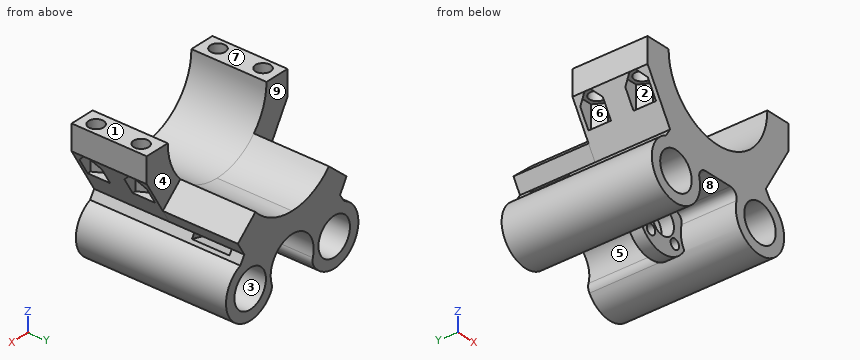
```python
from build123d import *

# Parameters (mm, degrees)
SKETCH1_R           = 11.5
SKETCH1_R_2         = 7.5
BOSS_EXTRUDE1_DEPTH = 30
FILLET1_R           = 3
SKETCH2_R           = 11.75
CUT_EXTRUDE3_DEPTH  = 3
SKETCH3_R           = 11.75
SKETCH3_R_2         = 5.25
SKETCH3_R_3         = 2
BOSS_EXTRUDE2_DEPTH = 5
SKETCH4_W           = 40
SKETCH4_H           = 60
BOSS_EXTRUDE3_DEPTH = 2
SKETCH5_R           = 10.25
CUT_EXTRUDE4_DEPTH  = 27
FILLET2_START       = -3
FILLET2_DEPTH       = 34
BOSS_EXTRUDE4_DEPTH = 30
BOSS_EXTRUDE5_DEPTH = 30
CUT_EXTRUDE5_DEPTH  = 15
SKETCH9_R           = 3
CUT_EXTRUDE6_DEPTH  = 10
CUT_EXTRUDE7_DEPTH  = 10


with BuildPart() as part:
    # Sketch1 → Boss-Extrude1 (new, symmetric)
    # profile 1 of 3: a face of its own
    with BuildSketch(Plane(origin=(0, 0, 0), x_dir=(1, 0, 0), z_dir=(0, 1, 0))):
        with Locations((-20, 0)):
            Circle(SKETCH1_R)
        with Locations(Location((-20, 0, 0), (0, 0, 270))):
            Circle(SKETCH1_R_2, mode=Mode.SUBTRACT)
    # profile 2 of 3: a face of its own
    with BuildSketch(Plane(origin=(0, 0, 0), x_dir=(1, 0, 0), z_dir=(0, 1, 0))):
        with Locations((20, 0)):
            Circle(SKETCH1_R)
        with Locations(Location((20, 0, 0), (0, 0, 270))):
            Circle(SKETCH1_R_2, mode=Mode.SUBTRACT)
    # profile 3 of 3: a face of its own
    with BuildSketch(Plane(origin=(0, 0, 0), x_dir=(1, 0, 0), z_dir=(0, 1, 0))):
        with BuildLine():
            ThreePointArc((-10.513167019, -6.5), (-14.638097353, -10.173494975), (-20, -11.5))
            Line((-20, -11.5), (20, -11.5))
            ThreePointArc((20, -11.5), (14.638097353, -10.173494975), (10.513167019, -6.5))
            Line((10.513167019, -6.5), (-10.513167019, -6.5))
        make_face()
    extrude(amount=BOSS_EXTRUDE1_DEPTH, both=True)

    # Fillet1
    fillet1_edges = [part.edges().sort_by_distance(p)[0] for p in [
        (-10.513167019, 0, 6.5),
        (10.513167019, 0, 6.5),
    ]]
    fillet(fillet1_edges, radius=FILLET1_R)

    # Sketch2 → Cut-Extrude3 (cut, symmetric)
    with BuildSketch(Plane(origin=(0, 0, 0), x_dir=(1, 0, 0), z_dir=(0, 1, 0))):
        Circle(SKETCH2_R)
    extrude(amount=CUT_EXTRUDE3_DEPTH, both=True, mode=Mode.SUBTRACT)

    # Sketch3 → Boss-Extrude2 (add)
    with BuildSketch(Plane(origin=(0, -3, 0), x_dir=(1, 0, 0), z_dir=(0, 1, 0))):
        Circle(SKETCH3_R)
        with Locations(Location((0, 0, 0), (0, 0, 270))):
            Circle(SKETCH3_R_2, mode=Mode.SUBTRACT)
        with Locations(Location((5.656854249, 5.656854249, 0), (0, 0, 270))):
            Circle(SKETCH3_R_3, mode=Mode.SUBTRACT)
        with Locations(Location((-5.656854249, 5.656854249, 0), (0, 0, 270))):
            Circle(SKETCH3_R_3, mode=Mode.SUBTRACT)
    extrude(amount=-BOSS_EXTRUDE2_DEPTH)

    # Sketch4 → Boss-Extrude3 (add)
    with BuildSketch(Plane.XY.offset(11.5)):
        Rectangle(SKETCH4_W, SKETCH4_H)
    extrude(amount=BOSS_EXTRUDE3_DEPTH)

    # Chamfer1
    # the kernel refuses this chamfer: 8 mm, written as the material it adds along each edge
    with BuildSketch(Plane(origin=(20, -30, 11.5), x_dir=(0.9777449098895067, 0, -0.20979726210120203), z_dir=(0, 1, 0))) as chamfer1_piece_1_section:
        with BuildLine():
            Line((5.051611198, 0.22627417), (-1.544518324, -6.369855352))
            Line((-1.544518324, -6.369855352), (-1.70095751, -6.33628779))
            ThreePointArc((-1.70095751, -6.33628779), (-0.843748586, -3.169588005), (-0.156439186, 0.033567562))
            Line((-0.156439186, 0.033567562), (0.033567562, 0.156439186))
            ThreePointArc((0.033567562, 0.156439186), (2.527924683, -0.095347808), (5.018043636, 0.382713356))
            Line((5.018043636, 0.382713356), (5.051611198, 0.22627417))
        make_face()
    chamfer1_piece_1 = extrude(amount=60, mode=Mode.PRIVATE)
    chamfer1_piece_1 = split(chamfer1_piece_1, bisect_by=Plane(origin=(20, -30, 13.5), z_dir=(0, 0, -1)), keep=Keep.TOP, mode=Mode.PRIVATE)
    add(chamfer1_piece_1)
    with BuildSketch(Plane(origin=(-20, -30, 11.5), x_dir=(-0.9777449098895067, 0, -0.20979726210120223), z_dir=(0, 1, 0))) as chamfer1_piece_2_section:
        with BuildLine():
            Line((5.051611198, -0.22627417), (-1.544518324, 6.369855352))
            Line((-1.544518324, 6.369855352), (-1.70095751, 6.33628779))
            ThreePointArc((-1.70095751, 6.33628779), (-0.843748586, 3.169588005), (-0.156439186, -0.033567562))
            Line((-0.156439186, -0.033567562), (0.033567562, -0.156439186))
            ThreePointArc((0.033567562, -0.156439186), (2.527924683, 0.095347808), (5.018043636, -0.382713356))
            Line((5.018043636, -0.382713356), (5.051611198, -0.22627417))
        make_face()
    chamfer1_piece_2 = extrude(amount=60, mode=Mode.PRIVATE)
    chamfer1_piece_2 = split(chamfer1_piece_2, bisect_by=Plane(origin=(-20, -30, 13.5), z_dir=(0, 0, -1)), keep=Keep.TOP, mode=Mode.PRIVATE)
    add(chamfer1_piece_2)

    # Sketch5 → Cut-Extrude4 (cut)
    with BuildSketch(Plane(origin=(0, 30, 0), x_dir=(1, 0, 0), z_dir=(0, 1, 0))):
        Circle(SKETCH5_R)
    extrude(amount=-CUT_EXTRUDE4_DEPTH, mode=Mode.SUBTRACT)

    # Fillet2: read off the stored shape, not the designer's step
    # Fillet2 outline → Fillet2 (cut)
    with BuildSketch(Plane(origin=(0, 0, 0), x_dir=(1, 0, 0), z_dir=(0, 1, 0)).offset(FILLET2_START)):
        with BuildLine():
            ThreePointArc((-9.833031798, 2.893783968), (-9.601199579, 3.588797381), (-9.3203125, 4.265474757))
            ThreePointArc((-9.3203125, 4.265474757), (-9.763069468, 5.239776072), (-10.294479167, 6.168700459))
            ThreePointArc((-10.294479167, 6.168700459), (-9.709438477, 4.581166738), (-9.833031798, 2.893783968))
        make_face()
        with BuildLine():
            ThreePointArc((10.294479167, 6.168700459), (9.763069468, 5.239776072), (9.3203125, 4.265474757))
            ThreePointArc((9.3203125, 4.265474757), (9.601199579, 3.588797381), (9.833031798, 2.893783968))
            ThreePointArc((9.833031798, 2.893783968), (9.709438477, 4.581166738), (10.294479167, 6.168700459))
        make_face()
    extrude(amount=FILLET2_DEPTH, mode=Mode.SUBTRACT)

    # Sketch6 → Boss-Extrude4 (add)
    with BuildSketch(Plane.XZ.offset(30)):
        with BuildLine():
            ThreePointArc((-23.5, 42), (0, 18.5), (23.5, 42))
            Line((23.5, 42), (33.5, 42))
            Line((33.5, 42), (33.5, 32))
            Line((33.5, 32), (22.769957826, 13.5))
            Line((22.769957826, 13.5), (-22.769957826, 13.5))
            Line((-22.769957826, 13.5), (-33.5, 32))
            Line((-33.5, 32), (-33.5, 42))
            Line((-33.5, 42), (-23.5, 42))
        make_face()
    extrude(amount=-BOSS_EXTRUDE4_DEPTH)

    # Sketch7 → Boss-Extrude5 (add)
    with BuildSketch(Plane(origin=(0, 0, 0), x_dir=(1, 0, 0), z_dir=(0, 1, 0))):
        with BuildLine():
            Line((0, -13.5), (0, -18.5))
            ThreePointArc((0, -18.5), (9.582977152, -20.542680761), (17.5, -26.315612859))
            Line((17.5, -26.315612859), (25.858213649, -18.824558077))
            Line((25.858213649, -18.824558077), (22.769957826, -13.5))
            Line((22.769957826, -13.5), (0, -13.5))
        make_face()
        with BuildLine():
            Line((-22.769957826, -13.5), (-25.858213649, -18.824558077))
            Line((-25.858213649, -18.824558077), (-17.5, -26.315612859))
            ThreePointArc((-17.5, -26.315612859), (-9.582977152, -20.542680761), (0, -18.5))
            Line((0, -18.5), (0, -13.5))
            Line((0, -13.5), (-22.769957826, -13.5))
        make_face()
    extrude(amount=BOSS_EXTRUDE5_DEPTH)

    # Sketch8 → Cut-Extrude5 (cut)
    with BuildSketch(Plane(origin=(0, 25, 0), x_dir=(1, 0, 0), z_dir=(0, 1, 0))):
        with BuildLine():
            Line((30.953633553, -14.257784453), (29.292282812, -15.746771207))
            ThreePointArc((29.292282812, -15.746771207), (0, -10.191127392), (-29.292282812, -15.746771207))
            Line((-29.292282812, -15.746771207), (-30.953633553, -14.257784453))
            ThreePointArc((-30.953633553, -14.257784453), (0, -8.191127392), (30.953633553, -14.257784453))
        make_face()
    extrude(amount=-CUT_EXTRUDE5_DEPTH, mode=Mode.SUBTRACT)

    # Sketch9 → Cut-Extrude6 (cut)
    with BuildSketch(Plane.XY.offset(42)):
        with Locations((29, -6)):
            Circle(SKETCH9_R)
        with Locations(Location((-29, -6, 0), (0, 0, 180))):
            Circle(SKETCH9_R)
        with Locations((-29, -24)):
            Circle(SKETCH9_R)
        with Locations(Location((29, -24, 0), (0, 0, 180))):
            Circle(SKETCH9_R)
    extrude(amount=-CUT_EXTRUDE6_DEPTH, mode=Mode.SUBTRACT)

    # Sketch10 → Cut-Extrude7 (cut)
    with BuildSketch(Plane.XY.offset(32)):
        Polygon((34.196152423, -6), (31.598076211, -1.5), (26.401923789, -1.5), (23.803847577, -6), (26.401923789, -10.5), (31.598076211, -10.5), align=None)
        Polygon((31.598076211, -19.5), (34.196152423, -24), (31.598076211, -28.5), (26.401923789, -28.5), (23.803847577, -24), (26.401923789, -19.5), align=None)
        Polygon((-34.196152423, -24), (-31.598076211, -28.5), (-26.401923789, -28.5), (-23.803847577, -24), (-26.401923789, -19.5), (-31.598076211, -19.5), align=None)
        Polygon((-31.598076211, -10.5), (-34.196152423, -6), (-31.598076211, -1.5), (-26.401923789, -1.5), (-23.803847577, -6), (-26.401923789, -10.5), align=None)
    extrude(amount=-CUT_EXTRUDE7_DEPTH, mode=Mode.SUBTRACT)


solid = part.part
```
The listing builds one solid part. Answer for the finished solid, in the listing's coordinates (mm). Face numbers are marked on the shaded views. A direction names the side the tool comes from. Round coordinates to 2 decimals unless told otherwise and drop trailing zeros. Write each loop counter-clockwise with the first axis right and the second up, starting at its lowest first coordinate (ties: lowest second). Pieces come first, ordered by that corner, then holes. Notation, with made-up numbers: (-34.5, -18.5) -> (-27.5, -18.5) arc R25 cw to (-27.5, -0.5) -> close; hole circle Ø3 at (-8.5, 25.25). An arc over 180 degrees is marked (long way). Answer as a JSON object with one key per item and string values. Group by question number.
Q1. Section D-D (z = 21) is taken. Write down the section's boundary in (x, y), plus the area to 3 significant figures.
Q2. Straight lines are drawn through the part: line 1 along Y through (x, z) = (29, 37); line 2 along X through (y, z) = (-18, 0); line 3 along X through (y, z) = (-7, 0). For each, find the intervals that lie inside material, in ascending order.
Q3. Determine the mould class of the marked faces 6, 7, 8 and 9 for opening direction Z: pulls with the +Z half, pulls with the -Z half, needs draft (parallel to the pull), parting line crosses it, or undercut.
Q4. Which of the six approach directions +Z, -Z, +X, -X, +Y, -Y give full straight-line access (tool end or side, diameter ignored) to the marked faces 1, 2, 3, 4 and 5?
Q5. Each of these flat-tipped pins is pushed along its axis until it touches: pin 1 Ø10 at (x, z) = (-21, 1.5) entering from -Y; pin 2 Ø16.5 at (x, z) = (0, 0) entering from +Y; pin 3 Ø8 at (y, z) = (10.5, -2) entering from -X; pin 4 Ø10 at (x, y) = (-25.5, 11.5) entering from -Z. Where does it stop, or does it pass through?
Q6. Section A-A (z = 34) is taken. Write down the section's boundary in (x, y).
Q7. Section B-B (x = -14) is taken. Write down the section's boundary in (y, z), plus the area to 3 significant figures.
Q8. Section C-C (y = 18) is taken. Write down the section's boundary in (x, z).
Check values:
{
 "1": {"outline": "(-27.12, -30) -> (-10.55, -30) -> (-10.55, 30) -> (-23.43, 30) -> (-23.43, 0) -> (-27.12, 0) -> close; (10.55, -30) -> (27.12, -30) -> (27.12, 0) -> (23.43, 0) -> (23.43, 30) -> (10.55, 30) -> close", "area": "1,770 mm^2"},
 "2": {"line 1": "-30 to -27, -21 to -9, -3 to 0", "line 2": "-31.5 to -27.5, -12.5 to -8.5, 8.5 to 12.5, 27.5 to 31.5", "line 3": "-31.5 to -27.5, -12.5 to -5.25, 5.25 to 12.5, 27.5 to 31.5"},
 "3": {"face 6": "undercut", "face 7": "pulls with the +Z half", "face 8": "pulls with the -Z half", "face 9": "needs draft"},
 "4": {"face 1": "+Z, +X, -X, +Y, -Y", "face 2": "none", "face 3": "+Y, -Y", "face 4": "+Z, +X, +Y", "face 5": "+Y"},
 "5": {"pin 1": "through", "pin 2": "y = -3", "pin 3": "x = -31.5", "pin 4": "z = -11.49"},
 "6": {"outline": "(-33.5, -30) -> (-22.1, -30) -> (-22.1, 0) -> (-33.5, 0) -> close; (22.1, -30) -> (33.5, -30) -> (33.5, 0) -> (22.1, 0) -> close; hole circle Ø6 at (-29, -24); hole circle Ø6 at (-29, -6); hole circle Ø6 at (29, -24); hole circle Ø6 at (29, -6)"},
 "7": {"outline": "(-30, -9.81) -> (30, -9.81) -> (30, -4.5) -> (-30, -4.5) -> close; (-30, 4.5) -> (30, 4.5) -> (30, 23.13) -> (-30, 23.13) -> close; hole (10, 9.4) -> (25, 9.4) -> (25, 11.43) -> (10, 11.43) -> close", "area": "1,410 mm^2"},
 "8": {"outline": "(-25.86, 18.82) -> (-22.77, 13.5) arc R80 ccw to (-1.03, 10.2) arc R10.25 cw to (1.03, 10.2) arc R80 ccw to (22.77, 13.5) -> (25.86, 18.82) -> (17.5, 26.32) arc R23.5 cw to (-17.5, 26.32) -> close; (-24.72, 10.49) arc R11.5 ccw (long way) to (-10.29, -6.17) arc R4 ccw to (-9.83, -2.89) arc R10.25 cw to (-5.87, 8.4) arc R82 cw to (-23.9, 11.75) -> close; (5.87, 8.4) arc R10.25 cw to (9.83, -2.89) arc R4 ccw to (10.29, -6.17) arc R11.5 ccw (long way) to (24.72, 10.49) -> (23.9, 11.75) arc R82 cw to start; hole circle Ø15 at (-20, 0); hole circle Ø15 at (20, 0)"}
}
